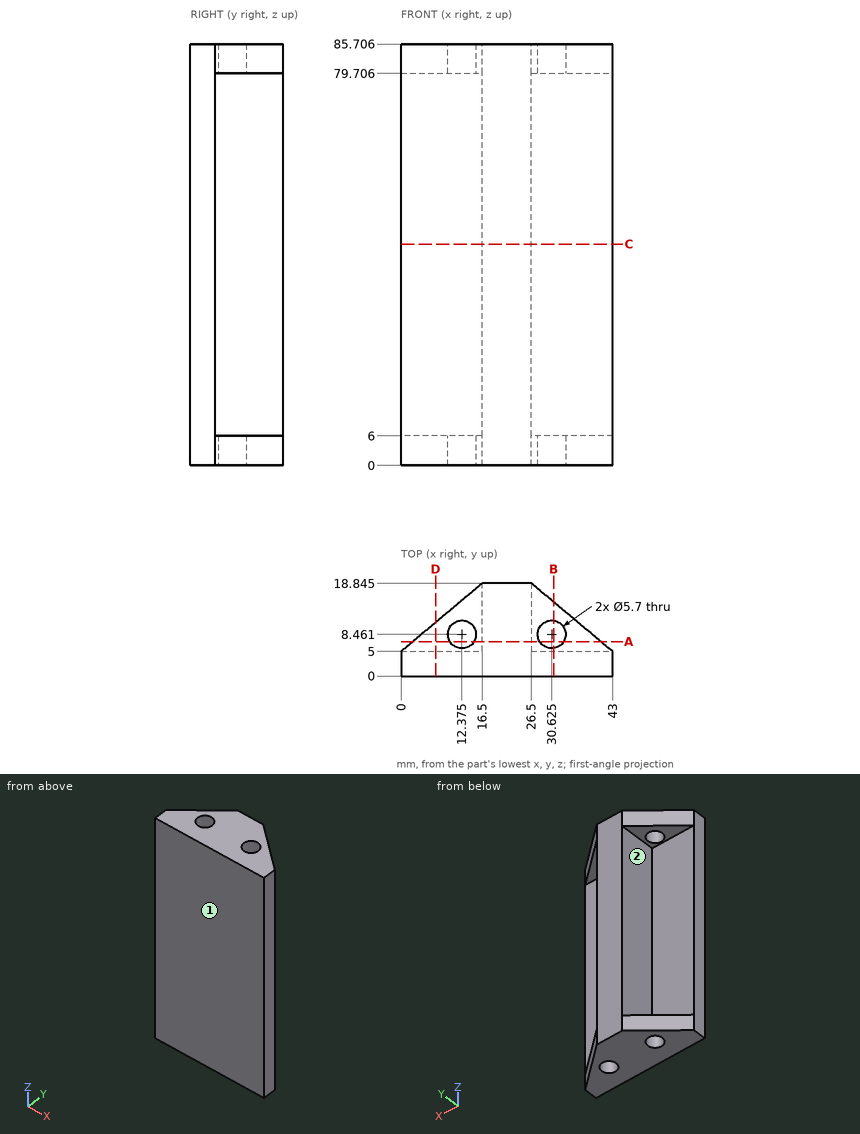
For this review, use the dimensioned drawing (mm, ordinates from the lowest corner) and the shaded views. A direction names the side the tool comes from. Round coordinates to 2 decimals unless told otherwise and drop trailing zeros. Loops run counter-clockwise (first coordinate to the right, second up) from the corner with the lowest first, then second, coordinate; pieces in that order, holes last. Notation, with made-up numbers: (85.25, 4.25) -> (105.25, 4.25) arc R18 ccw to (105.25, 16.25) -> close; hole circle Ø2 at (-16, -5). An arc over 180 degrees is marked (long way). Write item = value, one per line. Start each with the question number.
Item 1: To check wall thickness, follow L1, parallel to Z at x = 32.5, y = 5.75; L2, parallel to X at y = 5.75, z = 60; L3, parallel to Y at x = 38, z = 56.5. State the ranges of each line that lie inside material, in increasing order.
Item 2: Take a section at C-C on z = 45. Give the boundary of the cut face in (x, y) (1 decimal).
Item 3: Take a section at B-B on x = 31. Give the boundary of the cut face in (y, z).
Item 4: Take a section at D-D on x = 7. Give the boundary of the cut face in (y, z).
Item 5: For the marked faces 1 and 2, list the 3-axis set-ups (+Z, -Z, +X, -X, +Y, -Y) from which the entire face can be reached by the end or side of a thin tool; tool diameter is ignored.
Item 6: Take a section at A-A on y = 7. Give the boundary of the cut face in (x, z), plus the area to 3 significant figures.
Item 7: Insertion check: pin 1 (13 mm diameter, centred on x = 34, z = 46, fed in from +Y); pin 2 (8 mm diameter, centred on y = 14, z = 29, fed in from +X); pin 3 (4 mm diameter, centred on x = 38, y = 12, fed in from -Z); pin 4 (11 mm diameter, centred on y = 13, z = 36, fed in from -X). Each pin has a flat end and moves straight along its axis. Give the tip position at first contact, or say it passes through.
Result:
q1.L1 = 0 to 6, 79.71 to 85.71
q1.L2 = 16.5 to 26.5
q1.L3 = 0 to 5
q2.outline = (0, 0) -> (43, 0) -> (43, 5) -> (26.5, 5) -> (26.5, 18.8) -> (16.5, 18.8) -> (16.5, 5) -> (0, 5) -> close
q3.outline = (0, 0) -> (5.64, 0) -> (5.64, 6) -> (5, 6) -> (5, 79.71) -> (5.64, 79.71) -> (5.64, 85.71) -> (0, 85.71) -> close; (11.29, 0) -> (15.07, 0) -> (15.07, 6) -> (11.29, 6) -> close; (11.29, 79.71) -> (15.07, 79.71) -> (15.07, 85.71) -> (11.29, 85.71) -> close
q4.outline = (0, 0) -> (10.87, 0) -> (10.87, 6) -> (5, 6) -> (5, 79.71) -> (10.87, 79.71) -> (10.87, 85.71) -> (0, 85.71) -> close
q5.face_1 = +Z, -Z, +X, -X, -Y
q5.face_2 = -X, +Y
q6.outline = (2.38, 0) -> (9.93, 0) -> (9.93, 6) -> (2.38, 6) -> close; (2.38, 79.71) -> (9.93, 79.71) -> (9.93, 85.71) -> (2.38, 85.71) -> close; (14.82, 0) -> (28.18, 0) -> (28.18, 6) -> (26.5, 6) -> (26.5, 79.71) -> (28.18, 79.71) -> (28.18, 85.71) -> (14.82, 85.71) -> (14.82, 79.71) -> (16.5, 79.71) -> (16.5, 6) -> (14.82, 6) -> close; (33.07, 0) -> (40.62, 0) -> (40.62, 6) -> (33.07, 6) -> close; (33.07, 79.71) -> (40.62, 79.71) -> (40.62, 85.71) -> (33.07, 85.71) -> close
q6.area = 1,080 mm²
q7.pin_1 = 5
q7.pin_2 = 26.5
q7.pin_3 = through
q7.pin_4 = 16.5
